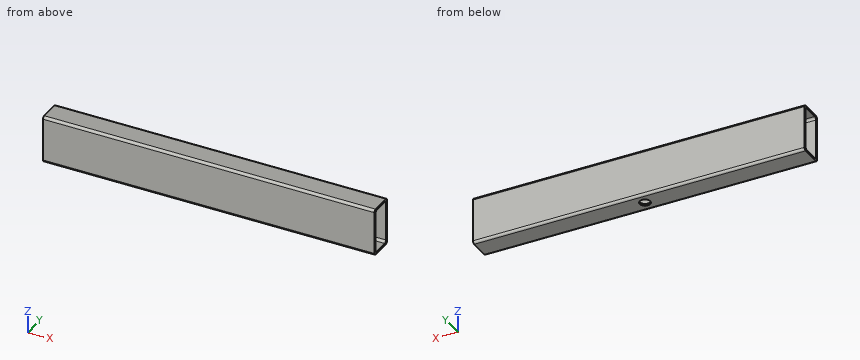
```python
from build123d import *

# Parameters (mm, degrees)
F0_W     = 700
F0_H     = 100
F1_DEPTH = 50
F2_T     = -4
F3_R     = 5
F5_D     = 22
F5_DEPTH = 4
F5_TIP   = 6.6094668093


with BuildPart() as f1:
    # F0 (on Front) → F1 (new body)
    with BuildSketch(Plane.XZ):
        Rectangle(F0_W, F0_H)
    extrude(amount=F1_DEPTH)

    # F2
    f2_openings = [f1.faces().sort_by_distance(p)[0] for p in [
        (-350, -25, 0),
        (350, -25, 0),
    ]]
    offset(amount=F2_T, openings=f2_openings)

    # F3
    f3_edges = [f1.edges().sort_by_distance(p)[0] for p in [
        (0, -4, 46),
        (0, -46, 46),
        (0, 0, 50),
        (0, -50, 50),
        (0, -4, -46),
        (0, -50, -50),
        (0, -46, -46),
        (0, 0, -50),
    ]]
    fillet(f3_edges, radius=F3_R)

    # F5
    with Locations(Plane(origin=(0, 0, -50), x_dir=(1, 0, 0), z_dir=(0, 0, -1))):
        with Locations((0, 25)):
            Hole(F5_D / 2, depth=F5_DEPTH)
            with Locations((0, 0, -(F5_DEPTH + F5_TIP / 2))):  # 118° drill point
                Cone(0, F5_D / 2, F5_TIP, mode=Mode.SUBTRACT)


solid = f1.part
```
Geometry: final body of the model. Coordinates: model frame, mm. Round coordinates to 2 decimals unless told otherwise and drop trailing zeros. Order: outer loops, then holes, each group sorted by start corner. A loop starts at its lowest first (then second) coordinate and runs counter-clockwise, first axis right, second up. Notation, with made-up numbers: (17.25, 42.25) - (75.25, 42.25) arc R13 cw to (75.25, 53.25) - close; hole circle Ø5 at (49.25, -36). An arc over 180 degrees is marked (long way). Write item = value, one per line. Start each with the question number.
Q1. Cut plane A-A on z = 35. Return the cut outline in (x, y), and give its area (3 significant figures).
Q2. Ray query, line 1 (Z direction, x = 82, y = -31.5); line 2 (Y direction, x = -70, z = -14); line 3 (Y direction, x = 0, z = -48.5). Return the intervals inside material, ascending. Write a range as from..to.
Q3. Cut plane D-D on x = 0. Return the cut outline in (y, z), and give its area (3 significant figures).
Q4. Cut plane B-B on y = -25. Return the cut outline in (x, z), and give its area (3 significant figures).
Q5. Cut plane C-C on x = -118.5. Return the cut outline in (y, z).
Outcome:
q1.outline = (-350, -50) - (350, -50) - (350, -46) - (-350, -46) - close; (-350, -4) - (350, -4) - (350, 0) - (-350, 0) - close
q1.area = 5,600 mm^2
q2.line_1 = -50..-46, 46..50
q2.line_2 = -50..-46, -4..0
q2.line_3 = -48.57..-36, -14..-1.43
q3.outline = (-50, -45) arc R5 ccw to (-45, -50) - (-36, -50) - (-36, -46) - (-41, -46) arc R5 cw to (-46, -41) - (-46, 41) arc R5 cw to (-41, 46) - (-9, 46) arc R5 cw to (-4, 41) - (-4, -41) arc R5 cw to (-9, -46) - (-14, -46) - (-14, -50) - (-5, -50) arc R5 ccw to (0, -45) - (0, 45) arc R5 ccw to (-5, 50) - (-45, 50) arc R5 ccw to (-50, 45) - close
q3.area = 1,050 mm^2
q4.outline = (-350, -50) - (-11, -50) - (-11, -46) - (-350, -46) - close; (-350, 46) - (350, 46) - (350, 50) - (-350, 50) - close; (11, -50) - (350, -50) - (350, -46) - (11, -46) - close
q4.area = 5,510 mm^2
q5.outline = (-50, -45) arc R5 ccw to (-45, -50) - (-5, -50) arc R5 ccw to (0, -45) - (0, 45) arc R5 ccw to (-5, 50) - (-45, 50) arc R5 ccw to (-50, 45) - close; hole (-46, -41) arc R5 ccw to (-41, -46) - (-9, -46) arc R5 ccw to (-4, -41) - (-4, 41) arc R5 ccw to (-9, 46) - (-41, 46) arc R5 ccw to (-46, 41) - close
